Here's how the part is built. I have some questions about the finished solid (model axes, mm). A direction names the side the tool comes from. Coordinates: 2 decimals unless noted, no trailing zeros. Write each loop counter-clockwise with the first axis right and the second up, starting at its lowest first coordinate (ties: lowest second). Pieces come first, ordered by that corner, then holes. Notation, with made-up numbers: (5.25, -19) -> (37.25, -19) arc R20 cw to (37.25, -3) -> close; hole circle Ø3 at (-4.75, -30). An arc over 180 degrees is marked (long way). Put each result on its own line as item: value. Start each with the question number.
Item 1: I want a section at D-D, the plane x = 4. List the corners of the cut face in (y, z) for me (3 decimals).
Item 2: For pin 1 (1.5 mm diameter, centred on x = -8.5, y = 0, fed in from +Z) (3 decimals); pin 2 (1.5 mm diameter, centred on x = -8.125, y = 0, fed in from -Z); pin 3 (6 mm diameter, centred on y = -2, z = 7, fed in from +X); pin 4 (3 mm diameter, centred on y = 4.5, z = 2, fed in from -X), each with a flat end and sliding along its axis, tell me the tip position at first contact or that it passes through.
Item 3: I want a section at C-C, the plane z = 4.25. List the corners of the cut face in (x, y) for me, then the cut area to 3 significant figures.
Item 4: I need wall thicknesses on line 1 (X direction, y = -8.2, z = 5); line 2 (X direction, y = -6, z = 10.25); line 3 (Z direction, x = -15, y = -9.05). Which ranges of each line are inside material? Lowest first, please. Write a range as [from, to].
Item 5: I want a section at A-A, the plane x = 0. List the corners of the cut face in (y, z) for me (3 decimals).
Item 6: I want a section at B-B, the plane y = -2.25. List the corners of the cut face in (x, z) for me (3 decimals), then the cut area to 3 significant figures.
Item 7: If we mould it in two halves opening along X, with no side actions, what happens to faces 1 (the face through (18, -9, 1)), 2 (the face through (0, -8, 7.175)), 3 (the face through (-8, 9, 9))? For each: released by +X, released by -X, zero draft, split by the parting line, or undercut.
Item 8: On a 3-axis mill with a long thin cutter (end or side, diameter ignored), from which of +Z, -Z, +X, -X, +Y, -Y can I reach the whole of each face in a straight line? I mean faces 4 (the face through (0, 6.25, 7)), 5 (the face through (-14, -7, 7)), 6 (the face through (2.7, 8, 11)), 7 (the face through (12.7, -7, 5.4)), 8 (the face through (10.2, -9, 13)). Say none if no direction works.
Autodesk Inventor part; units mm, degrees
ref_plane "YZ Plane" through (0, 0, 0) normal (1, 0, 0) x (0, 1, 0)
ref_plane "XZ Plane" through (0, 0, 0) normal (0, 1, 0) x (-1, 0, 0)
ref_plane "XY Plane" through (0, 0, 0) normal (0, 0, 1) x (1, 0, 0)
sketch "Sketch1" plane through (0, 0, 0) normal (0, 0, 1) x (1, 0, 0)
  line L0 (-6.25, 6.25) -> (6.25, 6.25)
  line L1 (6.25, 6.25) -> (6.25, -6.25)
  line L2 (6.25, -6.25) -> (-6.25, -6.25)
  line L3 (-6.25, -6.25) -> (-6.25, 6.25)
  line L4 (-10, 10) -> (10, 10)
  line L5 (10, 10) -> (10, -10)
  line L6 (10, -10) -> (-10, -10)
  line L7 (-10, -10) -> (-10, 10)
  line L8 (-10, 10) -> (10, -10) construction
  line L9 (10, 10) -> (-10, -10) construction
  dimension "d3" = 20
  dimension "d4" = 20
  dimension "d5" = 3.75
  dimension "d6" = 16.25
  dimension "d7" = 3.75
  dimension "d8" = 16.25
extrude "Extrusion1" add sketch "Sketch1" along normal blind 55
sketch "Sketch2" plane through (0, 0, 55) normal (0, 0, 1) x (1, 0, 0)
  line L0 (10, 10) -> (-10, 10)
  line L1 (-10, -10) -> (10, -10)
  line L2 (10, -10) -> (10, 10)
  line L3 (10, 10) -> (-10, 10)
  line L4 (-10, 10) -> (-10, -10)
  line L5 (-10, -10) -> (10, 10) construction
  line L6 (10, -10) -> (-10, 10) construction
  point P0 (0, 0)
extrude "Extrusion2" add sketch "Sketch2" along normal blind 3
sketch "Sketch3" plane through (0, 0, 55) normal (0, 0, -1) x (-1, 0, 0)
  circle A0 centre (0, 0) radius 4
  dimension "d13" = 8
extrude "Extrusion3" add sketch "Sketch3" along normal blind 14
sketch "Sketch4" plane through (10, -10, 0) normal (1, 0, 0) x (0, 0, -1)
  line L0 (0, 0) -> (-58, 0)
  line L1 (0, 0) -> (-10, 0)
  line L2 (-10, 0) -> (-10, 3)
  line L3 (-10, 3) -> (0, 3)
  line L4 (0, 3) -> (0, 0)
  line L5 (-58, 0) -> (-58, 20)
  line L6 (-58, 0) -> (-48, 0)
  line L7 (-48, 0) -> (-48, 3)
  line L8 (-48, 3) -> (-58, 3)
  line L9 (-58, 3) -> (-58, 0)
  point P0 (0, 10)
  dimension "d16" = 10
  dimension "d17" = 3
  dimension "d18" = 10
  dimension "d19" = 3
extrude "Extrusion4" add sketch "Sketch4" along normal blind 10
sketch "Sketch5" plane through (-10, -10, 0) normal (-1, 0, 0) x (0, 0, 1)
  line L0 (0, 0) -> (0, 20)
  line L1 (0, 3) -> (10, 3)
  line L2 (0, 0) -> (10, 0)
  line L3 (10, 0) -> (10, 3)
  line L4 (10, 3) -> (0, 3)
  line L5 (0, 3) -> (0, 0)
  line L6 (58, 20) -> (58, 0)
  line L7 (58, 0) -> (48, 0)
  line L8 (48, 0) -> (48, 3)
  line L9 (48, 3) -> (58, 3)
  line L10 (58, 3) -> (58, 0)
  point P0 (0, 10)
  dimension "d22" = 10
  dimension "d23" = 3
  dimension "d24" = 10
  dimension "d25" = 3
extrude "Extrusion5" add sketch "Sketch5" along normal blind 10
fillet "Fillet1" radius 5 12 edges at (-20, -8.5, 10) (-20, -8.5, 0) (-10, -8.5, 10) (-10, -8.5, 48) (-20, -8.5, 48) (-20, -8.5, 58) (20, -8.5, 0) (10, -8.5, 10) (20, -8.5, 10) (10, -8.5, 48) (20, -8.5, 48) (20, -8.5, 58)
sketch "Sketch6" plane through (10, -7, 15) normal (0, 1, 0) x (1, 0, 0)
  arc A0 (-25, 15) -> (-25, 5) centre (-25, 10) ccw
  circle A1 centre (-25, 10) radius 2
  arc A2 (5, 5) -> (5, 15) centre (5, 10) ccw
  circle A3 centre (5, 10) radius 2
  arc A4 (-25, -33) -> (-25, -43) centre (-25, -38) ccw
  circle A5 centre (-25, -38) radius 2
  arc A6 (5, -43) -> (5, -33) centre (5, -38) ccw
  circle A7 centre (5, -38) radius 2
  point P0 (-10, 15)
  dimension "d29" = 4
  dimension "d30" = 4
  dimension "d31" = 4
extrude "Extrusion6" cut sketch "Sketch6" against normal blind 10
fillet "Fillet2" radius 5 2 edges at (-10, 10, 29) (10, 10, 29)
sketch "Sketch7" plane through (-5, 10, 0) normal (0, 1, 0) x (1, 0, 0)
  arc A0 (7.7, -10) -> (2.3, -10) centre (5, -10) ccw
  line L0 (0, -58) -> (0, 0)
  arc A1 (2.3, -14.35) -> (7.7, -14.35) centre (5, -14.35) ccw
  line L1 (2.3, -14.35) -> (2.3, -10)
  line L2 (7.7, -14.35) -> (7.7, -10)
  point P0 (5, 0)
  dimension "d35" = 5.4
  dimension "d36" = 5
  dimension "d37" = 10
  dimension "d38" = 5.4
  dimension "d39" = 4.35
  dimension "d40" = 5
extrude "Extrusion7" cut sketch "Sketch7" against normal blind 10
sketch "Sketch8" plane through (-5, 10, 0) normal (0, 1, 0) x (1, 0, 0)
  line L0 (2.3, -10) -> (2.3, -14.35)
  line L1 (2.3, -12.175) -> (-5, -12.175)
  line L2 (-5, 0) -> (-5, -58)
  line L3 (-5, -15) -> (-5, -43)
  line L4 (-5, -12.175) -> (-5, -43)
  line L5 (-5, -43) -> (-15.8375, -43)
  line L6 (-15.8375, -43) -> (-15.3443, -61.3042)
  line L7 (-15.3443, -61.3042) -> (28.3034, -61.3042)
  line L8 (28.3034, -61.3042) -> (28.3034, -43)
  line L9 (15, -15) -> (15, -43)
  line L10 (28.3034, -43) -> (15, -43)
  line L11 (15, -43) -> (15, -12.175)
  line L12 (15, -12.175) -> (2.3, -12.175)
  point P0 (5, 0)
  dimension "d43" = 1.543
  dimension "d44" = 13.3034
  dimension "d45" = 18.3042
  dimension "d46" = 31.5804
extrude "Extrusion8" cut sketch "Sketch8" against normal blind 20
sketch "Sketch9" plane through (-5, 10, 12.175) normal (0, 0, 1) x (1, 0, 0)
  circle A0 centre (5, -18.125) radius 0.925
  circle A1 centre (13.125, -10) radius 0.925
  circle A2 centre (-3.125, -10) radius 0.925
  line L0 (-1.25, -3.75) -> (-1.25, -16.25)
  line L1 (11.25, -16.25) -> (11.25, -3.75)
  line L2 (-1.25, -16.25) -> (11.25, -16.25)
  point P0 (5, -10)
  dimension "d49" = 1.85
  dimension "d50" = 1.85
  dimension "d51" = 1.85
  dimension "d52" = 1.875
  dimension "d53" = 1.875
  dimension "d54" = 1.875
  dimension "d55" = 0
  dimension "d56" = 0
  dimension "d57" = 0
extrude "Extrusion9" cut sketch "Sketch9" against normal blind 5
sketch "Sketch10" plane through (-5, 10, 12.175) normal (0, 0, 1) x (1, 0, 0)
  line L0 (20, -20) -> (-10, -20)
  line L1 (15.2, 0) -> (-5.2, 0)
  line L2 (-5.2, 0) -> (-5.2, -20)
  line L3 (-5.2, -20) -> (15.2, -20)
  line L4 (15.2, -20) -> (15.2, 0)
  line L5 (15.2, 0) -> (-5.2, -20) construction
  line L6 (-5.2, 0) -> (15.2, -20) construction
  point P0 (5, -10)
  dimension "d60" = 20.4
extrude "Extrusion10" cut sketch "Sketch10" along normal blind 10
sketch "Sketch12" plane through (10, -7, 0) normal (1, 0, 0) x (0, 0, -1)
  line L0 (0, 17) -> (0, 12)
  line L1 (0, 17) -> (-6, 17)
  line L2 (-12.175, 17) -> (0, 17)
  line L3 (0, 17) -> (0, 7)
  line L4 (0, 13.25) -> (0, 0.75)
  line L5 (-6, 17) -> (0, 7)
  dimension "d68" = 6
  dimension "d69" = 10
extrude "Extrusion12" cut sketch "Sketch12" against normal blind 20
properties part number "15 slot pinhuls klijn"
Calculated:
1. outline: (-10, 0) -> (-6.25, 0) -> (-6.25, 12.175) -> (-10, 12.175) -> close; (6.25, 3.75) -> (10, 6) -> (10, 12.175) -> (6.25, 12.175) -> close
2. pin 1: stops at z = 12.175
2. pin 2: stops at z = 0
2. pin 3: stops at x = 10
2. pin 4: stops at x = -10
3. outline: (-19.94, -10) -> (-16.85, -10) -> (-16.85, -7) -> (-19.94, -7) -> close; (-13.15, -10) -> (13.15, -10) -> (13.15, -7) -> (10, -7) -> (10, 5) arc R5 ccw to (9.55, 7.08) -> (-9.55, 7.08) arc R5 ccw to (-10, 5) -> (-10, -7) -> (-13.15, -7) -> close; (16.85, -10) -> (19.94, -10) -> (19.94, -7) -> (16.85, -7) -> close; hole (-6.25, -6.25) -> (6.25, -6.25) -> (6.25, 6.25) -> (-6.25, 6.25) -> close
3. area: 222 mm2
4. line 1: x = [-20, -17], [-13, 13], [17, 20]
4. line 2: x = [-10, -6.25], [6.25, 10]
4. line 3: z = [0, 3], [7, 10]
5. outline: (-10, 0) -> (-6.25, 0) -> (-6.25, 12.175) -> (-7.2, 12.175) -> (-7.2, 7.175) -> (-9.05, 7.175) -> (-9.05, 12.175) -> (-10, 12.175) -> close; (6.25, 3.75) -> (10, 6) -> (10, 7.3) -> (6.25, 7.3) -> close
6. outline: (-10, 0) -> (-6.25, 0) -> (-6.25, 12.175) -> (-10, 12.175) -> close; (6.25, 0) -> (10, 0) -> (10, 12.175) -> (6.25, 12.175) -> close
6. area: 91.3 mm2
7. face 1: released by +X
7. face 2: undercut
7. face 3: released by -X
8. face 4: +Z, -Z
8. face 5: +Z, -Z, -X, +Y
8. face 6: +Z, +Y
8. face 7: +Z, -Z, +X, +Y
8. face 8: +Z, +Y, -Y
